Verification items for the finished model (mm, model axes). Round coordinates to 2 decimals unless told otherwise and drop trailing zeros. Loops run counter-clockwise (first coordinate to the right, second up) from the corner with the lowest first, then second, coordinate; pieces in that order, holes last. Notation, with made-up numbers: (28.5, 57) - (49.5, 57) arc R17 cw to (49.5, 77) - close; hole circle Ø4 at (-15.5, -2). An arc over 180 degrees is marked (long way). Use CSV: the item, a comma, the result in double quotes.
```python
from build123d import *

# Parameters (mm, degrees)
CUT_EXTRUDE_START   = -9
SKETCH_2_R          = 0.5
CUT_EXTRUDE_1_DEPTH = 10
SKETCH_3_R          = 2.5
CUT_EXTRUDE_2_DEPTH = 3


with BuildPart() as part:
    # 草图1 → 旋转1 (revolve)
    with BuildSketch(Plane.XY):
        Polygon((0, 0), (5, 0), (0, 10), align=None)
    revolve(axis=Axis((0, 0, 0), (0, 1, 0)))

    # 草图2 → 切除-拉伸1 (cut)
    with BuildSketch(Plane.XZ.offset(CUT_EXTRUDE_START)):
        Circle(SKETCH_2_R)
    extrude(amount=-CUT_EXTRUDE_1_DEPTH, mode=Mode.SUBTRACT)

    # 草图3 → 切除-拉伸2 (cut)
    with BuildSketch(Plane.XZ):
        Circle(SKETCH_3_R)
    extrude(amount=-CUT_EXTRUDE_2_DEPTH, mode=Mode.SUBTRACT)


solid = part.part
```
1) Cross-section at B-B, the plane z = 0. Record the cut outline in (x, y), then the cut area to 3 significant figures.
Returned:
outline,"(-5, 0) - (-2.5, 0) - (-2.5, 3) - (2.5, 3) - (2.5, 0) - (5, 0) - (0.5, 9) - (-0.5, 9) - close"
area,"34.5 mm²"
2) Mould release check, pull along Z, two halves, no side actions. Record for faces 1 (the face through (-0.54, 1.48, -2.44)), 2 (the face through (0, 6, 2)), 3 (the face through (-2, 0, 2)), 4 (the face through (0, 3, 0)): +Z half, -Z half, draft (parallel to the pull), parting line (faces both ways), or undercut.
Returned:
face 1,"undercut"
face 2,"parting line"
face 3,"draft"
face 4,"undercut"
3) Thickness scan on probe 1 along Z at (x, y) = (0, 2.2); probe 2 along X at (y, z) = (0.5, -1.5); probe 3 along Z at (x, y) = (0, 0.85) (3 decimals). Record the ranges inside material, lowest first. Write a range as [from, to].
Returned:
probe 1,"z = [-3.9, -2.5], [2.5, 3.9]"
probe 2,"x = [-4.51, -2], [2, 4.51]"
probe 3,"z = [-4.575, -2.5], [2.5, 4.575]"
4) Gauge pin test, flat ends, axial feed: pin 1 Ø2 at (y, z) = (2, 4) entering from -X; pin 2 Ø4 at (x, z) = (0, 0) entering from -Y; pin 3 Ø5 at (x, y) = (2, 4.5) entering from +Z; pin 4 Ø1 at (y, z) = (6.5, -2.5) entering from +X. Record the tip position at first contact, or that the pin passes through.
Returned:
pin 1,"stops at x = -2.87"
pin 2,"stops at y = 3"
pin 3,"stops at z = 3.77"
pin 4,"passes through"
5) Cross-section at D-D, the plane y = 3.25. Record the cut outline in (x, z) (3 decimals).
Returned:
outline,"circle Ø6.75 at (0, 0)"
6) Cross-section at A-A, the plane x = 0. Record the cut outline in (y, z).
Returned:
outline,"(0, -5) - (9, -0.5) - (9, 0.5) - (0, 5) - (0, 2.5) - (3, 2.5) - (3, -2.5) - (0, -2.5) - close"
7) Cross-section at C-C, the plane y = 6.5. Record the cut outline in (x, z).
Returned:
outline,"circle Ø3.5 at (0, 0)"
